from build123d import *

# Parameters (mm, degrees)
F0_W     = 10
F0_H     = 10
F1_DEPTH = 144
F2_W     = 10
F2_H     = 5
F3_DEPTH = 10


with BuildPart() as f1:
    # F0 (on Front) → F1 (new body)
    with BuildSketch(Plane.XZ):
        Rectangle(F0_W, F0_H)
    extrude(amount=F1_DEPTH)

    # F2 (on face) → F3 (cut)
    with BuildSketch(Plane.YZ.offset(5)):
        with Locations((-139, 2.5)):
            Rectangle(F2_W, F2_H)
        with Locations((-5, 2.5)):
            Rectangle(F2_W, F2_H)
    extrude(amount=-F3_DEPTH, mode=Mode.SUBTRACT)


solid = f1.part
The listing builds one solid part. Answer for the finished solid, in the listing's coordinates (mm). A direction names the side the tool comes from. Coordinates: 2 decimals unless noted, no trailing zeros. Order: outer loops, then holes, each group sorted by start corner. A loop starts at its lowest first (then second) coordinate and runs counter-clockwise, first axis right, second up. Notation, with made-up numbers: (9.5, -23.75) -> (64.5, -23.75) arc R21 cw to (64.5, -15.75) -> close; hole circle Ø1 at (38.25, -31). An arc over 180 degrees is marked (long way). Answer in a Markdown table with one row per item. Add a question column.
Item 1: Find section A-A (x = -2.5). Write down the section's boundary in (y, z), then the cut area to 3 significant figures.
Item 2: Each of these flat-tipped pins is pushed along its axis until it touches: P1, Ø1, axis at x = -0.5, z = -1.5, coming from the +Y side; P2, Ø1.5, axis at x = -0.5, z = 3.5, coming from the +Y side; P3, Ø1.5, axis at x = -1.5, z = 3.5, coming from the -Y side. Where does it stop, or does it pass through?
Item 3: Find the intervals of material crossed by L1, parallel to Y at x = 0, z = 3, in increasing order. Write a range as from..to.
Item 4: Which of the six approach directions +Z, -Z, +X, -X, +Y, -Y give full straight-line access (tool end or side, diameter ignored) to faces 1 (the face through (0, -134, 2)), 2 (the face through (0, -5, 0)), 3 (the face through (0, 0, -2))?
Item 5: Find section B-B (z = 3). Write down the section's boundary in (x, y).
Result set:
| question | item | result |
|---|---|---|
| 1 | outline | (-144, -5) -> (0, -5) -> (0, 0) -> (-10, 0) -> (-10, 5) -> (-134, 5) -> (-134, 0) -> (-144, 0) -> close |
| 1 | area | 1,340 mm² |
| 2 | P1 | stops at y = 0 |
| 2 | P2 | stops at y = -10 |
| 2 | P3 | stops at y = -134 |
| 3 | L1 | y = -134..-10 |
| 4 | face 1 | +Z, +X, -X, -Y |
| 4 | face 2 | +Z, +X, -X, +Y |
| 4 | face 3 | +Z, -Z, +X, -X, +Y |
| 5 | outline | (-5, -134) -> (5, -134) -> (5, -10) -> (-5, -10) -> close |
